Here's how the part is built. I have some questions about the finished solid (model axes, mm). A direction names the side the tool comes from. Give positions to 0.01 mm unless a question says otherwise; leave off trailing zeros. Loops run counter-clockwise (first coordinate to the right, second up) from the corner with the lowest first, then second, coordinate; pieces in that order, holes last.
Q1. Suppose I cut it at D-D (y = 34). List the corners of the cut face in (x, z) for me (1 decimal).
Q2. I need wall thicknesses on probe 1 along Z at (x, y) = (0, -100); probe 2 along Y at (x, z) = (3, 25); probe 3 along Y at (x, z) = (8, 120.5). Which ranges of each line are inside material? Lowest first, please.
Q3. Suppose I cut it at C-C (z = 0). List the corners of the cut face in (x, y) for me, and give its area (3 significant figures).
Q4. I'm going to push flat-ended pins straight in: P1, Ø18, axis at x = 0, z = 0, coming from the +Y side; P2, Ø10, axis at x = 104, z = 77.5, coming from the +Y side; P3, Ø3, axis at x = 1.5, y = -61, coming from the -Z side. Where does each tip first touch, or does it pass through?
Q5. Suppose I cut it at B-B (z = 90). List the corners of the cut face in (x, y) for me.
Q6. Suppose I cut it at A-A (x = 5). List the corners of the cut face in (y, z) for me.
Q7. Thinking about a two-plate mould opening in Z: for faces 1 (the face through (-14.362, 62.611, -11.012)), 2 (the face through (82.96, -130.13, 66.71)), 3 (the face through (14.233, 64.389, 4.482)), which applies, pulls with the +Z half, pulls with the -Z half, needs draft (parallel to the pull), parting line crosses it, or undercut?
Q8. For faces 4 (the face through (-23.17, -130.13, -10.41)), 5 (the face through (3, 127, 15)), 6 (the face through (0, 0, 0)), 7 (the face through (14.233, -65.83, 4.482)), which set-ups out of +Z, -Z, +X, -X, +Y, -Y let a thin tool reach every point of the face, with its end or its side?
```python
from build123d import *

# Parameters (mm, degrees)
F0_R     = 18.0975
F0_R_2   = 14.9225
F1_DEPTH = 127
F3_DEPTH = 6.35
F5_DEPTH = 6.35


with BuildPart() as f1:
    # F0 (on Front) → F1 (new body, symmetric)
    with BuildSketch(Plane.XZ):
        Circle(F0_R)
        Circle(F0_R_2, mode=Mode.SUBTRACT)
    extrude(amount=F1_DEPTH, both=True)

    # F2 (on Front) → F3 (join)
    with BuildSketch(Plane.XZ):
        Polygon((0, -25.4), (25.4, -25.4), (25.4, 228.6), (0, 228.6), (-25.4, 228.6), (-25.4, -25.4), align=None)
    extrude(amount=F3_DEPTH)

    # F4 (on face) → F5 (join)
    with BuildSketch(Plane.XZ.offset(127)):
        Polygon((217.916464, 73.590317), (207.18196, 96.610535), (196.447456, 119.630752), (-33.754722, 12.285714), (-23.020218, -10.734504), (-12.285714, -33.754722), align=None)
    extrude(amount=F5_DEPTH)


solid = f1.part
```
Solutions:
1. outline: circle Ø36.2 at (0, 0); hole circle Ø29.8 at (0, 0)
2. probe 1: z = -18.1 to -14.92, 14.92 to 18.1
2. probe 2: y = -133.35 to -127, -6.35 to 0
2. probe 3: y = -6.35 to 0
3. outline: (-28.03, -133.35) - (60.1, -133.35) - (60.1, -127) - (18.1, -127) - (18.1, -6.35) - (25.4, -6.35) - (25.4, 0) - (18.1, 0) - (18.1, 127) - (14.92, 127) - (14.92, 0) - (-14.92, 0) - (-14.92, 127) - (-18.1, 127) - (-18.1, 0) - (-25.4, 0) - (-25.4, -6.35) - (-18.1, -6.35) - (-18.1, -127) - (-28.03, -127) - close; hole (-14.92, -127) - (14.92, -127) - (14.92, -6.35) - (-14.92, -6.35) - close
3. area: 2,450 mm2
4. P1: stops at y = 0
4. P2: stops at y = -127
4. P3: stops at z = -18.1
5. outline: (-25.4, -6.35) - (25.4, -6.35) - (25.4, 0) - (-25.4, 0) - close; (132.9, -133.35) - (210.26, -133.35) - (210.26, -127) - (132.9, -127) - close
6. outline: (-133.35, -25.69) - (-127, -25.69) - (-127, -17.39) - (-6.35, -17.39) - (-6.35, -25.4) - (0, -25.4) - (0, -17.39) - (127, -17.39) - (127, -14.06) - (0, -14.06) - (0, 14.06) - (127, 14.06) - (127, 17.39) - (0, 17.39) - (0, 228.6) - (-6.35, 228.6) - (-6.35, 17.39) - (-127, 17.39) - (-127, 30.36) - (-133.35, 30.36) - close; hole (-127, -14.06) - (-6.35, -14.06) - (-6.35, 14.06) - (-127, 14.06) - close
7. face 1: parting line crosses it
7. face 2: pulls with the +Z half
7. face 3: undercut
8. face 4: -Z, -X, -Y
8. face 5: +Z, -Z, +X, -X, +Y
8. face 6: +Y
8. face 7: none
